from build123d import *

# Parameters (mm, degrees)
F0_W     = 150
F0_H     = 250
F1_DEPTH = 55
F2_W     = 118
F2_H     = 175
F3_DEPTH = 55.001
F4_R     = 5
F5_T     = -2.5
F6_W     = 145
F6_H     = 49.9277314544
F7_DEPTH = 50


with BuildPart() as f1:
    # F0 (on Front) → F1 (new body)
    with BuildSketch(Plane.XZ):
        with Locations((75, 125)):
            Rectangle(F0_W, F0_H)
    extrude(amount=F1_DEPTH)

    # F2 (on face) → F3 (cut, through all)
    with BuildSketch(Plane.XZ.offset(55)):
        with Locations((75, 142.5)):
            Rectangle(F2_W, F2_H)
    extrude(amount=-F3_DEPTH, mode=Mode.SUBTRACT)

    # F4
    f4_edges = [f1.edges().sort_by_distance(p)[0] for p in [
        (16, -27.5, 230),
        (134, -27.5, 230),
        (134, -27.5, 55),
        (16, -27.5, 55),
    ]]
    fillet(f4_edges, radius=F4_R)

    # F5
    f5_openings = [f1.faces().sort_by_distance(p)[0] for p in [
        (16, -27.5, 142.5),
        (17.464466, -27.5, 56.464466),
        (75, -27.5, 55),
        (132.535534, -27.5, 56.464466),
        (134, -27.5, 142.5),
        (17.464466, -27.5, 228.535534),
        (75, -27.5, 230),
        (132.535534, -27.5, 228.535534),
    ]]
    offset(amount=F5_T, openings=f5_openings)

    # F6 (on face) → F7 (join, through all)
    with BuildSketch(Plane.XZ.offset(2.5)):
        with Locations((75, 27.4638657272)):
            Rectangle(F6_W, F6_H)
    extrude(amount=F7_DEPTH)


solid = f1.part
Read the model definition and answer for the solid it produces. Units are mm, in the model's axes. A direction names the side the tool comes from. Round coordinates to 2 decimals unless told otherwise and drop trailing zeros. Loops run counter-clockwise (first coordinate to the right, second up) from the corner with the lowest first, then second, coordinate; pieces in that order, holes last.
Q1. Section A-A on z = 107 is taken. Write down the section's boundary in (x, y), and give its area (3 significant figures).
Q2. Section B-B on y = -15 is taken. Write down the section's boundary in (x, z).
Q3. Section C-C on x = 93.5 is taken. Write down the section's boundary in (y, z).
Q4. Which of the six approach directions +Z, -Z, +X, -X, +Y, -Y give full straight-line access (tool end or side, diameter ignored) to faces 1 (the face through (18, -54, 56)), 2 (the face through (15.6, -52.5, 172.1)), 3 (the face through (74, -27, 0))?
Q5. Section D-D on z = 235 is taken. Write down the section's boundary in (x, y), and give its area (3 significant figures).
Q6. Consider probe 1 along X at (y, z) = (-42, 190); probe 2 along Z at (x, y) = (99, -35); probe 3 along Y at (x, z) = (142, 57). Determine where each line is inside the solid, lowest interval first.
Q7. Determine the mould class of faces 4 (the face through (150, -27, 123)), 5 (the face through (141, 0, 99)), 6 (the face through (74, -27, 52.428)) for opening direction Y: released by +Y, released by -Y, zero draft, split by the parting line, or undercut.
Output:
1. outline: (0, -55) - (16, -55) - (16, -52.5) - (2.5, -52.5) - (2.5, -2.5) - (16, -2.5) - (16, 0) - (0, 0) - close; (134, -55) - (150, -55) - (150, 0) - (134, 0) - (134, -2.5) - (147.5, -2.5) - (147.5, -52.5) - (134, -52.5) - close
1. area: 410 mm2
2. outline: (0, 0) - (150, 0) - (150, 250) - (0, 250) - close; hole (2.5, 52.43) - (147.5, 52.43) - (147.5, 247.5) - (2.5, 247.5) - close
3. outline: (-55, 0) - (0, 0) - (0, 55) - (-2.5, 55) - (-2.5, 52.43) - (-52.5, 52.43) - (-52.5, 55) - (-55, 55) - close; (-55, 230) - (-52.5, 230) - (-52.5, 247.5) - (-2.5, 247.5) - (-2.5, 230) - (0, 230) - (0, 250) - (-55, 250) - close
4. face 1: +Y, -Y
4. face 2: none
4. face 3: -Z, +X, -X, +Y, -Y
5. outline: (0, -55) - (150, -55) - (150, 0) - (0, 0) - close; hole (2.5, -52.5) - (147.5, -52.5) - (147.5, -2.5) - (2.5, -2.5) - close
5. area: 1,000 mm2
6. probe 1: x = 0 to 2.5, 147.5 to 150
6. probe 2: z = 0 to 52.43, 247.5 to 250
6. probe 3: y = -55 to -52.5, -2.5 to 0
7. face 4: zero draft
7. face 5: released by +Y
7. face 6: undercut
